```python
from build123d import *

# Parameters (mm, degrees)
SKETCH2_W           = 71.12
SKETCH2_H           = 15.875
BOSS_EXTRUDE1_DEPTH = 35.56
FILLET1_R           = 3.96875
SKETCH3_R           = 1.905
REVOLVE1_ANGLE      = 90


with BuildPart() as part:
    # Sketch2 → Boss-Extrude1 (new body)
    with BuildSketch(Plane(origin=(0, 0, 0), x_dir=(1, 0, 0), z_dir=(0, 1, 0))):
        Rectangle(SKETCH2_W, SKETCH2_H)
    extrude(amount=BOSS_EXTRUDE1_DEPTH)

    # Fillet1
    fillet1_edges = [part.edges().sort_by_distance(p)[0] for p in [
        (35.56, 17.78, 7.9375),
        (35.56, 17.78, -7.9375),
    ]]
    fillet(fillet1_edges, radius=FILLET1_R)

    # Sketch3 → Revolve1 (revolve)
    with BuildSketch(Plane(origin=(0, 35.56, 0), x_dir=(1, 0, 0), z_dir=(0, 1, 0))):
        with Locations((31.59125, -3.96875)):
            Circle(SKETCH3_R)
        with Locations((31.59125, 3.96875)):
            Circle(SKETCH3_R)
    revolve(axis=Axis((35.56, 35.56, -7.9375), (0, 0, -1)), revolution_arc=REVOLVE1_ANGLE)


solid = part.part
```
Here's how the part is built. I have some questions about the finished solid (model axes, mm). A direction names the side the tool comes from. Coordinates: 2 decimals unless noted, no trailing zeros. Write each loop counter-clockwise with the first axis right and the second up, starting at its lowest first coordinate (ties: lowest second). Pieces come first, ordered by that corner, then holes. Notation, with made-up numbers: (-14, -1.5) -> (38, -1.5) arc R17 ccw to (38, 2.5) -> close; hole circle Ø3 at (-33.75, -20). An arc over 180 degrees is marked (long way). Use a Markdown table: item, result. Add a question column.
(1) If we section it at C-C, the plane z = 0: Write out the boundary of the cut face in (x, y), and give its area (3 significant figures).
(2) If we section it at B-B, the plane x = 0.5: Write out the boundary of the cut face in (y, z).
(3) I'm going to push a flat-ended pin straight in: P1, Ø6, axis at x = -11, z = 4.5, coming from the +Y side. Where does the tip first touch, or does it pass through?
(4) For faces 1 (the cylindrical face through (34.43, 18.03, -6.74)), 2 (the cylindrical face through (34.367, 18.029, 6.806)), 3 (the flat face through (-2, 18, 7.938)), which set-ups out of +Z, -Z, +X, -X, +Y, -Y let a thin tool reach every point of the face, with its end or its side?
(5) If we section it at A-A, the plane z = -5: Write out the boundary of the cut face in (x, y).
(6) Please list where these lines run through material, in increasing order: line 1 (Y direction, x = -31, z = 2); line 2 (X direction, y = 30, z = 4.25); line 3 (X direction, y = 21, z = 6.5).
Outcome:
| question | item | result |
|---|---|---|
| 1 | outline | (-35.56, 0) -> (35.56, 0) -> (35.56, 35.56) -> (-35.56, 35.56) -> close |
| 1 | area | 2,530 mm^2 |
| 2 | outline | (0, -7.94) -> (35.56, -7.94) -> (35.56, 7.94) -> (0, 7.94) -> close |
| 3 | P1 | stops at y = 35.56 |
| 4 | face 1 | -Z, +X, -Y |
| 4 | face 2 | +Z, +X, -Y |
| 4 | face 3 | +Z, +X, -X, +Y, -Y |
| 5 | outline | (-35.56, 0) -> (35.42, 0) -> (35.42, 35.56) -> (33.19, 35.56) arc R2.37 cw to (35.56, 37.93) -> (35.56, 41.13) arc R5.57 ccw to (29.99, 35.56) -> (-35.56, 35.56) -> close |
| 6 | line 1 | y = 0 to 35.56 |
| 6 | line 2 | x = -35.56 to 35.55 |
| 6 | line 3 | x = -35.56 to 34.65 |
